Part model, mm, in its own coordinate system. A direction names the side the tool comes from. Coordinates: 2 decimals unless noted, no trailing zeros. Write each loop counter-clockwise with the first axis right and the second up, starting at its lowest first coordinate (ties: lowest second). Pieces come first, ordered by that corner, then holes. Notation, with made-up numbers: (-21, 56) -> (-5, 56) arc R21 cw to (-5, 67) -> close; hole circle Ø9 at (-39.75, -34). An arc over 180 degrees is marked (long way). Write item = value, one per line. Start each with the question number.
Q1. Band-saw the part on B-B, the plane x = 6.75. List the corners of the cut face in (y, z), plus the area to 3 significant figures.
Q2. Band-saw the part on D-D, the plane y = 2.2. List the corners of the cut face in (x, z).
Q3. Tool access for faces 5 (the flat face through (0, 1, 4)), 6 (the flat face through (0, 2.5, 0)), 7 (the cylindrical face through (-9.93, 3.867, 7.46)): list every direction of +Z, -Z, +X, -X, +Y, -Y with a clear straight run to the whole face (end or side of a thin tool).
Q4. Band-saw the part on A-A, the plane z = 0. List the corners of the cut face in (x, y), plus the area to 3 significant figures.
Q5. Band-saw the part on C-C, the plane y = 4.1. List the corners of the cut face in (x, z).
Q6. Pin check, flat tips, straight feed: P1, Ø1.2, axis at y = 2.5, z = 6, coming from the +X side; P2, Ø2.5, axis at x = -4, z = -0.5, coming from the +Y side. Stop position of each tip, or through.
Q7. Probe line 1 (X direction, y = 1.7, z = 0); line 2 (Y direction, x = 8.25, z = 6); line 3 (Z direction, x = -12.25, y = 2.4). List the from-to ranges inside material, lowest first.
Q8. Pull direction X, two halves, no side cores. Call faces 1 (the flat face through (-15, 2, 2)), 2 (the flat face through (10.07, 0.246, 4.986)), 3 (the flat face through (5, 1, 6)), 4 (the flat face through (-5, 1, 6)): released by +X, released by -X, zero draft, split by the parting line, or undercut.
from build123d import *

# Parameters (mm, degrees)
SKETCH1_W                       = 30
SKETCH1_H                       = 8
SKETCH1_R                       = 2.5
BOSS_EXTRUDE1_DEPTH             = 2.5
BOSS_EXTRUDE2_REACH             = 17
SKETCH2_R                       = 1.25
BOSS_EXTRUDE2_DIRECTION_2_REACH = 17
SKETCH4_W                       = 10
SKETCH4_H                       = 4
CUT_EXTRUDE2_DEPTH              = 5.5


with BuildPart() as part:
    # Sketch1 → Boss-Extrude1 (new body)
    with BuildSketch(Plane(origin=(0, 0, 0), x_dir=(1, 0, 0), z_dir=(0, 1, 0))):
        Rectangle(SKETCH1_W, SKETCH1_H)
        with Locations((-7.5, 0)):
            Circle(SKETCH1_R, mode=Mode.SUBTRACT)
        with Locations((7.5, 0)):
            Circle(SKETCH1_R, mode=Mode.SUBTRACT)
    extrude(amount=BOSS_EXTRUDE1_DEPTH)

    # Boss-Extrude2: up to this face of the body (flat: up to its plane)
    boss_extrude2_end = Plane(part.part.faces().sort_by_distance((15, 1.25, 0))[0])
    # Sketch2 → Boss-Extrude2 (add, up to the picked face)
    with BuildSketch(Plane(origin=(0, 0, 0), x_dir=(0, 0, -1), z_dir=(1, 0, 0)), mode=Mode.PRIVATE) as boss_extrude2_sk1:
        with BuildLine():
            Line((-4, 2.5), (-4, 0))
            Line((-4, 0), (-6, 0.5))
            ThreePointArc((-6, 0.5), (-7.414213562, 3.914213562), (-4, 2.5))
        make_face()
        with Locations((-6, 2.5)):
            Circle(SKETCH2_R, mode=Mode.SUBTRACT)
    boss_extrude2_tool1 = split(extrude(boss_extrude2_sk1.sketch, amount=BOSS_EXTRUDE2_REACH, mode=Mode.PRIVATE), bisect_by=boss_extrude2_end, keep=Keep.BOTH, mode=Mode.PRIVATE)
    add(boss_extrude2_tool1.solids().sort_by_distance((0, 1.25, 4.060208))[0])

    # Boss-Extrude2 direction 2: up to this face of the body (flat: up to its plane)
    boss_extrude2_direction_2_end = Plane(part.part.faces().sort_by_distance((-15, 1.25, 0))[0])
    # Sketch2 → Boss-Extrude2 direction 2 (add, up to the picked face)
    with BuildSketch(Plane(origin=(0, 0, 0), x_dir=(0, 0, -1), z_dir=(1, 0, 0)), mode=Mode.PRIVATE) as boss_extrude2_direction_2_sk1:
        with BuildLine():
            Line((-4, 2.5), (-4, 0))
            Line((-4, 0), (-6, 0.5))
            ThreePointArc((-6, 0.5), (-7.414213562, 3.914213562), (-4, 2.5))
        make_face()
        with Locations((-6, 2.5)):
            Circle(SKETCH2_R, mode=Mode.SUBTRACT)
    boss_extrude2_direction_2_tool1 = split(extrude(boss_extrude2_direction_2_sk1.sketch, amount=-BOSS_EXTRUDE2_DIRECTION_2_REACH, mode=Mode.PRIVATE), bisect_by=boss_extrude2_direction_2_end, keep=Keep.BOTH, mode=Mode.PRIVATE)
    add(boss_extrude2_direction_2_tool1.solids().sort_by_distance((0, 1.25, 4.060208))[0])

    # Sketch4 → Cut-Extrude2 (cut, through all)
    with BuildSketch(Plane(origin=(0, 0, 0), x_dir=(1, 0, 0), z_dir=(0, 1, 0))):
        with Locations((0, -6)):
            Rectangle(SKETCH4_W, SKETCH4_H)
    extrude(amount=CUT_EXTRUDE2_DEPTH, mode=Mode.SUBTRACT)


solid = part.part
Ans:
q1.outline = (0, -4) -> (2.5, -4) -> (2.5, -2.38) -> (0, -2.38) -> close; (0, 2.38) -> (2.5, 2.38) -> (2.5, 4) arc R2 ccw (long way) to (0.5, 6) -> (0, 4) -> close; hole circle Ø2.5 at (2.5, 6)
q1.area = 17.1 mm2
q2.outline = (-15, -4) -> (15, -4) -> (15, 4.79) -> (5, 4.79) -> (5, 4) -> (-5, 4) -> (-5, 4.79) -> (-15, 4.79) -> close; (-15, 7.21) -> (-5, 7.21) -> (-5, 7.98) -> (-15, 7.98) -> close; (5, 7.21) -> (15, 7.21) -> (15, 7.98) -> (5, 7.98) -> close; hole circle Ø5 at (-7.5, 0); hole circle Ø5 at (7.5, 0)
q3.face_5 = +Z, +Y, -Y
q3.face_6 = -Z, +X, -X, +Y
q3.face_7 = +X, -X
q4.outline = (-15, 0) -> (-10, 0) -> (-10, 2.5) -> (-15, 2.5) -> close; (-5, 0) -> (5, 0) -> (5, 2.5) -> (-5, 2.5) -> close; (10, 0) -> (15, 0) -> (15, 2.5) -> (10, 2.5) -> close
q4.area = 50.0 mm2
q5.outline = (-15, 4.8) -> (-5, 4.8) -> (-5, 7.2) -> (-15, 7.2) -> close; (5, 4.8) -> (15, 4.8) -> (15, 7.2) -> (5, 7.2) -> close
q6.P1 = through
q6.P2 = 2.5
q7.line_1 = -15 to -10, -5 to 5, 10 to 15
q7.line_2 = 0.5 to 1.25, 3.75 to 4.5
q7.line_3 = -4 to 4.75, 7.25 to 8
q8.face_1 = released by -X
q8.face_2 = zero draft
q8.face_3 = undercut
q8.face_4 = undercut
